```python
from build123d import *

# Parameters (mm, degrees)
F0_R     = 11
F1_DEPTH = 5


with BuildPart() as f1:
    # F0 (on Top) → F1 (new body)
    with BuildSketch(Plane.XY):
        with BuildLine():
            ThreePointArc((-13.124451, -15.082959), (-16.514327, -6.328217), (-24.916067, -2.139242))
            ThreePointArc((-24.916067, -2.139242), (-37.427089, -21.505605), (-14.386187, -20.669831))
            ThreePointArc((-14.386187, -20.669831), (-13.443808, -17.946747), (-13.124451, -15.082959))
        make_face()
        with Locations((-26.124451, -15.082959)):
            Circle(F0_R, mode=Mode.SUBTRACT)
        with BuildLine():
            ThreePointArc((39.124451, -15.082959), (34.944886, -5.533093), (25.093693, -2.123888))
            ThreePointArc((25.093693, -2.123888), (14.910958, -8.505911), (14.310672, -20.508326))
            ThreePointArc((14.310672, -20.508326), (28.901218, -27.782942), (39.124451, -15.082959))
        make_face()
        with Locations((26.124451, -15.082959)):
            Circle(F0_R, mode=Mode.SUBTRACT)
        with BuildLine():
            ThreePointArc((10.605395, 22.647568), (12.386891, 26.220677), (13, 30.165918))
            ThreePointArc((13, 30.165918), (-3.860209, 42.579571), (-10.707506, 22.793719))
            ThreePointArc((-10.707506, 22.793719), (-0.089144, 17.166224), (10.605395, 22.647568))
        make_face()
        with Locations((0, 30.165918)):
            Circle(F0_R, mode=Mode.SUBTRACT)
        with BuildLine():
            ThreePointArc((10.605395, 22.647568), (-0.089144, 17.166224), (-10.707506, 22.793719))
            ThreePointArc((-10.707506, 22.793719), (-14.883109, 8.658271), (-24.916067, -2.139242))
            ThreePointArc((-24.916067, -2.139242), (-16.514327, -6.328217), (-13.124451, -15.082959))
            ThreePointArc((-13.124451, -15.082959), (-13.443808, -17.946747), (-14.386187, -20.669831))
            ThreePointArc((-14.386187, -20.669831), (-0.056728, -17.218286), (14.310672, -20.508326))
            ThreePointArc((14.310672, -20.508326), (14.910958, -8.505911), (25.093693, -2.123888))
            ThreePointArc((25.093693, -2.123888), (14.939837, 8.560015), (10.605395, 22.647568))
        make_face()
        Circle(F0_R, mode=Mode.SUBTRACT)
    extrude(amount=F1_DEPTH)


solid = f1.part
```
Verification items for the finished model (mm, model axes). Coordinates: 2 decimals unless noted, no trailing zeros. Loops run counter-clockwise (first coordinate to the right, second up) from the corner with the lowest first, then second, coordinate; pieces in that order, holes last. Notation, with made-up numbers: (67.25, -31.5) - (78.25, -31.5) arc R15 cw to (78.25, -6.5) - close; hole circle Ø3 at (89, 61). An arc over 180 degrees is marked (long way). Answer as a JSON object with one key per item and string values.
(1) Go/stop test with flat-tipped pins: pin 1 Ø3 at (x, z) = (-28, 0.5) entering from -Y; pin 2 Ø1.5 at (y, z) = (24, 3.5) entering from -X. Record where each tip stops, or that it passes through.
Response:
{"pin 1": "stops at y = -28.08", "pin 2": "stops at x = -11.82"}
(2) Scan lines: line 1 along Y through (x, z) = (0, 1.6); line 2 along Y through (x, z) = (-9.5, 0.95); line 3 along Y through (x, z) = (-20.5, 0.5). Record each from-to range of solid material in increasing order.
Response:
{"line 1": "y = -17.22 to -11, 11 to 19.17, 41.17 to 43.17", "line 2": "y = -18.69 to -5.55, 5.55 to 24.62, 35.71 to 39.04", "line 3": "y = -26.8 to -24.54, -5.63 to 1.43"}
(3) Cross-section at B-B, the plane x = 0. Record the boundary of the cut face in (y, z), then the cut area to 3 significant figures.
Response:
{"outline": "(-17.22, 0) - (-11, 0) - (-11, 5) - (-17.22, 5) - close; (11, 0) - (19.17, 0) - (19.17, 5) - (11, 5) - close; (41.17, 0) - (43.17, 0) - (43.17, 5) - (41.17, 5) - close", "area": "81.9 mm²"}
(4) Mould release check, pull along X, two halves, no side actions. Record for faces 1 (the cylindrical face through (31.2, -24.84, 2.46)), 2 (the cylindrical face through (-2.38, -10.74, 2.46)), 3 (the flat face through (-3, -11, 0)): pulls with the +X half, pulls with the -X half, needs draft (parallel to the pull), parting line crosses it, or undercut.
Response:
{"face 1": "undercut", "face 2": "undercut", "face 3": "needs draft"}
(5) Cross-section at C-C, the plane z = 1.1. Record the boundary of the cut face in (x, y), then the cut area to 3 significant figures.
Response:
{"outline": "(-24.92, -2.14) arc R13 ccw (long way) to (-14.39, -20.67) arc R32.22 cw to (14.31, -20.51) arc R13 ccw to (39.12, -15.08) arc R13 ccw to (25.09, -2.12) arc R32.22 cw to (10.61, 22.65) arc R13 ccw (long way) to (-10.71, 22.79) arc R32.22 cw to start; hole circle Ø22 at (-26.12, -15.08); hole circle Ø22 at (0, 0); hole circle Ø22 at (0, 30.17); hole circle Ø22 at (26.12, -15.08)", "area": "1,240 mm²"}
(6) Cross-section at D-D, the plane x = -19. Record the boundary of the cut face in (y, z), then the cut area to 3 significant figures.
Response:
{"outline": "(-25.96, 0) - (-23.46, 0) - (-23.46, 5) - (-25.96, 5) - close; (-6.7, 0) - (2.98, 0) - (2.98, 5) - (-6.7, 5) - close", "area": "60.9 mm²"}
(7) Cross-section at A-A, the plane y = 0. Record the boundary of the cut face in (x, z).
Response:
{"outline": "(-22.08, 0) - (-11, 0) - (-11, 5) - (-22.08, 5) - close; (11, 0) - (22.21, 0) - (22.21, 5) - (11, 5) - close"}
